Autodesk Inventor part; units mm, degrees
ref_plane "YZ Plane" through (0, 0, 0) normal (1, 0, 0) x (0, 1, 0)
ref_plane "XZ Plane" through (0, 0, 0) normal (0, 1, 0) x (-1, 0, 0)
ref_plane "XY Plane" through (0, 0, 0) normal (0, 0, 1) x (1, 0, 0)
sketch "Sketch1" plane through (0, 0, 0) normal (0, 1, 0) x (-1, 0, 0)
  line L0 (0, 60) -> (0, 57.25) construction
  line L1 (0, 60) -> (-2.75, 60) construction
  line L2 (0, -60) -> (-2.75, -60) construction
  line L3 (-115.25, -55) -> (-7.75, -55)
  line L4 (-5, -55) -> (-5, -52.25) construction
  line L5 (-5, 55) -> (-7.75, 55) construction
  line L6 (-115.25, 55) -> (-115.25, 60)
  line L7 (-115.25, -60) -> (-115.25, -55)
  arc A0 (-5, 52.25) -> (-7.75, 55) centre (-7.75, 52.25) ccw
  arc A1 (-7.75, -55) -> (-5, -52.25) centre (-7.75, -52.25) ccw
  arc A2 (0, 57.25) -> (-2.75, 60) centre (-2.75, 57.25) ccw
  arc A3 (-2.75, -60) -> (0, -57.25) centre (-2.75, -57.25) ccw
  line L8 (0, 57.25) -> (0, -57.25)
  line L9 (-2.75, 60) -> (-115.25, 60)
  line L10 (0, -57.25) -> (0, -60) construction
  line L11 (-2.75, -60) -> (-115.25, -60)
  line L12 (-5, -52.25) -> (-5, 52.25)
  line L13 (-7.75, -55) -> (-5, -55) construction
  line L14 (-5, 52.25) -> (-5, 55) construction
  line L15 (-7.75, 55) -> (-115.25, 55)
  arc A4 (-2.75, 60) -> (0, 57.25) centre (-2.75, 57.25) ccw construction
  arc A5 (-7.75, 55) -> (-5, 52.25) centre (-7.75, 52.25) ccw construction
  arc A6 (0, -57.25) -> (-2.75, -60) centre (-2.75, -57.25) ccw construction
  arc A7 (-5, -52.25) -> (-7.75, -55) centre (-7.75, -52.25) ccw construction
  point P0 (0, 0)
  point P1 (0, 0)
  dimension "d4" = 5
  dimension "d6" = 115.25
  dimension "d8" = 115.25
  dimension "d9" = 5
  dimension "d10" = 5
  dimension "d11" = 120
  dimension "d12" = 55
  dimension "d13" = 5.5
extrude "Plate1" add sketch "Sketch1" against normal blind 2
equation "\"d9\" = d4"
equation "\"d10\" = d4"
equation "\"d11\" = Ширина_крепления_корпуса"
equation "\"d5\" = Thickness"
equation "\"BendReliefWidth\" = Thickness"
equation "\"BendReliefDepth\" = 0.5 * Thickness"
equation "\"CornerReliefSize\" = 4 * Thickness"
equation "\"MinimumRemnant\" = 2 * Thickness"
equation "\"TransitionRadius\" = BendRadius"
equation "\"JacobiRadiusSize\" = BendRadius"
equation "\"GapSize\" = Thickness"
properties part number "Опоры на кожухе 2" material "Stainless Steel"
Here's how the part is built. I have some questions about the finished solid (model axes, mm). A direction names the side the tool comes from. Coordinates: 2 decimals unless noted, no trailing zeros. Loops run counter-clockwise (first coordinate to the right, second up) from the corner with the lowest first, then second, coordinate; pieces in that order, holes last.
1. If we mould it in two halves opening along Z, with no side actions, what happens to faces 1 (the flat face through (2, 0, 0)), 2 (the cylindrical face through (5.78, -0.99, 54.17)), 3 (the cylindrical face through (0.83, -0.99, -59.22))? For each: pulls with the +Z half, pulls with the -Z half, needs draft (parallel to the pull), parting line crosses it, or undercut.
2. I need wall thicknesses on L1, parallel to Z at x = 56, y = -1.35; L2, parallel to X at y = -0.45, z = -34; L3, parallel to X at y = -1, z = -54. Which ranges of each line are inside material? Lowest first, please.
3. For faces 4 (the cylindrical face through (5.83, -0.99, -54.22)), 5 (the cylindrical face through (0.78, -0.99, 59.17)), which set-ups out of +Z, -Z, +X, -X, +Y, -Y let a thin tool reach every point of the face, with its end or its side?
4. Imagine slicing it at B-B, the plane y = -1.4. Please give me the cut outline in (x, z).
5. For P1, Ø0.6, axis at y = -1, z = 0.5, coming from the +X side, with a flat end and sliding along its axis, tell me the tip position at first contact or that it passes through.
6. Imagine slicing it at C-C, the plane z = -5. Please give me the cut outline in (x, y), and give its area (3 significant figures).
7. Imagine slicing it at A-A, the plane x = 26. Please give me the cut outline in (y, z).
Taken from the geometry:
1. face 1: needs draft
1. face 2: undercut
1. face 3: pulls with the -Z half
2. L1: z = -60 to -55, 55 to 60
2. L2: x = 0 to 5
2. L3: x = 0 to 5.63
3. face 4: +X, +Y, -Y
3. face 5: +Z, -X, +Y, -Y
4. outline: (0, -57.25) arc R2.75 ccw to (2.75, -60) - (115.25, -60) - (115.25, -55) - (7.75, -55) arc R2.75 cw to (5, -52.25) - (5, 52.25) arc R2.75 cw to (7.75, 55) - (115.25, 55) - (115.25, 60) - (2.75, 60) arc R2.75 ccw to (0, 57.25) - close
5. P1: stops at x = 5
6. outline: (0, -2) - (5, -2) - (5, 0) - (0, 0) - close
6. area: 10.0 mm2
7. outline: (-2, -60) - (0, -60) - (0, -55) - (-2, -55) - close; (-2, 55) - (0, 55) - (0, 60) - (-2, 60) - close
